from build123d import *

# Parameters (mm, degrees)
SKETCH1_W                    = 55
SKETCH1_H                    = 30
BOSS_EXTRUDE1_DEPTH          = 12
SKETCH2_R                    = 8.5
CUT_EXTRUDE1_DEPTH           = 34.544746235
SKETCH4_W                    = 12
SKETCH4_H                    = 5
CUT_EXTRUDE2_DEPTH           = 5
FILLET1_R                    = 2
SKETCH5_W                    = 12
SKETCH5_H                    = 5
CUT_EXTRUDE3_DEPTH           = 3
FILLET2_R                    = 5
BOSS_EXTRUDE3_DEPTH          = 8
F_3_0MM_DOWEL_HOLE1_D        = 3
SKETCH10_W                   = 8
SKETCH10_H                   = 8
BOSS_EXTRUDE4_DEPTH          = 2
F_2_0_2_DIAMETER_HOLE1_D     = 2
F_2_0_2_DIAMETER_HOLE1_DEPTH = 10
F_2_0_2_DIAMETER_HOLE1_TIP   = 0.600860619


with BuildPart() as part:
    # Sketch1 → Boss-Extrude1 (new body)
    with BuildSketch(Plane(origin=(0, 0, 0), x_dir=(1, 0, 0), z_dir=(0, 1, 0))):
        Rectangle(SKETCH1_W, SKETCH1_H)
    extrude(amount=BOSS_EXTRUDE1_DEPTH)

    # Sketch2 → Cut-Extrude1 (cut, through all)
    with BuildSketch(Plane(origin=(0, 12, 0), x_dir=(1, 0, 0), z_dir=(0, 1, 0))):
        with Locations(Location((-13.12, 0, 0), (0, 0, 270))):
            Circle(SKETCH2_R)
        with Locations(Location((13.12, 0, 0), (0, 0, 270))):
            Circle(SKETCH2_R)
    extrude(amount=-CUT_EXTRUDE1_DEPTH, mode=Mode.SUBTRACT)

    # Sketch4 → Cut-Extrude2 (cut)
    with BuildSketch(Plane.XZ):
        with Locations((0, -7.5)):
            Rectangle(SKETCH4_W, SKETCH4_H)
    extrude(amount=-CUT_EXTRUDE2_DEPTH, mode=Mode.SUBTRACT)

    # Fillet1
    fillet1_edges = [part.edges().sort_by_distance(p)[0] for p in [
        (-6, 2.5, -10),
        (-6, 2.5, -5),
        (6, 2.5, -5),
        (6, 2.5, -10),
    ]]
    fillet(fillet1_edges, radius=FILLET1_R)

    # Sketch5 → Cut-Extrude3 (cut)
    with BuildSketch(Plane.XZ):
        with Locations((0, 12.5)):
            Rectangle(SKETCH5_W, SKETCH5_H)
    extrude(amount=-CUT_EXTRUDE3_DEPTH, mode=Mode.SUBTRACT)

    # Fillet2
    fillet2_edges = [part.edges().sort_by_distance(p)[0] for p in [
        (27.5, 6, 15),
        (-27.5, 6, 15),
        (-27.5, 6, -15),
        (27.5, 6, -15),
    ]]
    fillet(fillet2_edges, radius=FILLET2_R)

    # Sketch6 → Boss-Extrude3 (add)
    with BuildSketch(Plane.XZ):
        with BuildLine():
            Line((25.5, 10), (25.5, -10))
            ThreePointArc((25.5, -10), (24.621320344, -12.121320344), (22.5, -13))
            Line((22.5, -13), (-22.5, -13))
            ThreePointArc((-22.5, -13), (-24.621320344, -12.121320344), (-25.5, -10))
            Line((-25.5, -10), (-25.5, 10))
            ThreePointArc((-25.5, 10), (-24.621320344, 12.121320344), (-22.5, 13))
            Line((-22.5, 13), (-8, 13))
            Line((-8, 13), (-6, 13))
            Line((-6, 13), (-6, 15))
            Line((-6, 15), (-22.5, 15))
            ThreePointArc((-22.5, 15), (-26.035533906, 13.535533906), (-27.5, 10))
            Line((-27.5, 10), (-27.5, -10))
            ThreePointArc((-27.5, -10), (-26.035533906, -13.535533906), (-22.5, -15))
            Line((-22.5, -15), (22.5, -15))
            ThreePointArc((22.5, -15), (26.035533906, -13.535533906), (27.5, -10))
            Line((27.5, -10), (27.5, 10))
            ThreePointArc((27.5, 10), (26.035533906, 13.535533906), (22.5, 15))
            Line((22.5, 15), (6, 15))
            Line((6, 15), (6, 13))
            Line((6, 13), (8, 13))
            Line((8, 13), (22.5, 13))
            ThreePointArc((22.5, 13), (24.621320344, 12.121320344), (25.5, 10))
        make_face()
    extrude(amount=BOSS_EXTRUDE3_DEPTH)

    # Ø3.0mm Dowel Hole1 (through all)
    with Locations(Plane.ZY.offset(27.5)):
        with Locations((0, -5)):
            Hole(F_3_0MM_DOWEL_HOLE1_D / 2)

    # Sketch10 → Boss-Extrude4 (add)
    with BuildSketch(Plane.ZY.offset(-25.5)):
        with Locations((0, -4)):
            Rectangle(SKETCH10_W, SKETCH10_H)
        Polygon((2.771281292, -5), (1.385640646, -2.6), (-1.385640646, -2.6), (-2.771281292, -5), (-1.385640646, -7.4), (1.385640646, -7.4), align=None, mode=Mode.SUBTRACT)
    boss_extrude4 = extrude(amount=BOSS_EXTRUDE4_DEPTH)

    # Mirror1: Boss-Extrude4 across plane
    add(boss_extrude4.mirror(Plane(origin=(0, 0, 0), x_dir=(0, 0, 1), z_dir=(1, 0, 0))))

    # Ø2.0 (2) Diameter Hole1
    with Locations(Plane(origin=(0, 0, 0), x_dir=(-1, 0, 0), z_dir=(0, -1, 0))):
        with Locations((-21.425, 8.7), (21.425, 8.7), (21.425, -8.7), (-21.425, -8.7)):
            Hole(F_2_0_2_DIAMETER_HOLE1_D / 2, depth=F_2_0_2_DIAMETER_HOLE1_DEPTH)
            with Locations((0, 0, -(F_2_0_2_DIAMETER_HOLE1_DEPTH + F_2_0_2_DIAMETER_HOLE1_TIP / 2))):  # 118° drill point
                Cone(0, F_2_0_2_DIAMETER_HOLE1_D / 2, F_2_0_2_DIAMETER_HOLE1_TIP, mode=Mode.SUBTRACT)


solid = part.part
Geometry check sheet. Reference: the model listing, model coordinates, mm. A direction names the side the tool comes from. Coordinates: 2 decimals unless noted, no trailing zeros. Loops run counter-clockwise (first coordinate to the right, second up) from the corner with the lowest first, then second, coordinate; pieces in that order, holes last. Notation, with made-up numbers: (-9.75, 28) - (47.25, 28) arc R20 cw to (47.25, 59) - close; hole circle Ø7 at (-7.75, 3). An arc over 180 degrees is marked (long way). Use one line per item in the form item = value. Start each with the question number.
Item 1: Mould release check, pull along X, two halves, no side actions. Record for faces 4 (the face through (-27.5, 2, 0)), 5 (the face through (25, -2.6, 0)), 6 (the face through (26.514, -3.513, 0.195)), 7 (the face through (25.5, -3, 0)): +X half, -X half, draft (parallel to the pull), parting line (faces both ways), or undercut.
Item 2: Section check C-C, the plane y = -1. Enter the section's corners in (x, z).
Item 3: Section check D-D, the plane z = -6. Enter the section's corners in (x, y).
Item 4: Tool access check on faces 1 (the face through (25, -7.4, 0)), 2 (the face through (0, 3, 13)), 3 (the face through (22.35, 5.07, 9.08)). Record the directions out of +Z, -Z, +X, -X, +Y, -Y that give a thin tool (end or side, any length) a straight path to the whole face; none if there is none.
Item 5: Section check A-A, the plane z = 0. Give the number of separate pieces and of enclosed holes in the cut face, and give its area (3 significant figures).
Item 6: Section check B-B, the plane x = -13.12. Enter the section's corners in (y, z), and give its area (3 significant figures).
Item 7: Gauge pin test, flat ends, axial feed: pin 1 (2.5 mm diameter, centred on x = -1, z = 13, fed in from -Y); pin 2 (2 mm diameter, centred on x = -24.5, y = -5.5, fed in from -Z); pin 3 (12 mm diameter, centred on x = -13.5, z = -3, fed in from -Y). Record the tip position at first contact, or that the pin passes through.
Item 8: Thickness scan on probe 1 along X at (y, z) = (7.5, -8.7) (3 decimals); probe 2 along X at (y, z) = (-2.25, 1.5); probe 3 along Z at (x, y) = (-12.5, -4.25). Record the ranges inside material, lowest first.
Computed:
q1.face_4 = -X half
q1.face_5 = undercut
q1.face_6 = draft
q1.face_7 = undercut
q2.outline = (-27.5, -10) arc R5 ccw to (-22.5, -15) - (22.5, -15) arc R5 ccw to (27.5, -10) - (27.5, 10) arc R5 ccw to (22.5, 15) - (6, 15) - (6, 13) - (22.5, 13) arc R3 cw to (25.5, 10) - (25.5, 4) - (23.5, 4) - (23.5, -4) - (25.5, -4) - (25.5, -10) arc R3 cw to (22.5, -13) - (-22.5, -13) arc R3 cw to (-25.5, -10) - (-25.5, -4) - (-23.5, -4) - (-23.5, 4) - (-25.5, 4) - (-25.5, 10) arc R3 cw to (-22.5, 13) - (-6, 13) - (-6, 15) - (-22.5, 15) arc R5 ccw to (-27.5, 10) - close
q3.outline = (-27.5, -8) - (-25.5, -8) - (-25.5, 0) - (-19.14, 0) - (-19.14, 12) - (-27.5, 12) - close; (-7.1, 0) - (-5.73, 0) - (-5.73, 5) - (5.73, 5) - (5.73, 0) - (7.1, 0) - (7.1, 12) - (-7.1, 12) - close; (19.14, 0) - (25.5, 0) - (25.5, -8) - (27.5, -8) - (27.5, 12) - (19.14, 12) - close
q4.face_1 = none
q4.face_2 = +Z, -Y
q4.face_3 = -Y
q5.separate_pieces = 5
q5.enclosed_holes = 0
q5.area = 285 mm2
q6.outline = (-8, -15) - (12, -15) - (12, -8.5) - (0, -8.5) - (0, -13) - (-8, -13) - close; (-8, 13) - (0, 13) - (0, 8.5) - (12, 8.5) - (12, 15) - (-8, 15) - close
q6.area = 188 mm2
q7.pin_1 = 3
q7.pin_2 = -14.9
q7.pin_3 = 0
q8.probe_1 = -27.5 to -22.425, -20.425 to 20.425, 22.425 to 27.5
q8.probe_2 = -27.5 to -23.5, 23.5 to 27.5
q8.probe_3 = -15 to -13, 13 to 15
